```python
from build123d import *

# Parameters (mm, degrees)
CHAMFER_1_SIZE            = 0.2
FILLET_1_R                = 0.2
HOLE_WIZARD_4_0_4_1_D     = 4
HOLE_WIZARD_4_0_4_1_DEPTH = 2.5
HOLE_WIZARD_4_0_4_1_TIP   = 1.201721238
CUT_EXTRUDE_1_DEPTH       = 2.5
FILLET_2_R                = 0.2


with BuildPart() as part:
    # 草图1 → 旋转1 (revolve)
    with BuildSketch(Plane.XY):
        Polygon((0, 0), (0, 4.25), (5, 4.25), (5, 2.5), (40, 2.5), (40, 0), align=None)
    revolve(axis=Axis((0, 0, 0), (1, 0, 0)))

    # 倒角1
    chamfer_1_edges = [part.edges().sort_by_distance(p)[0] for p in [
        (40, -2.5, 0),
    ]]
    chamfer(chamfer_1_edges, length=CHAMFER_1_SIZE)

    # 圆角1
    fillet_1_edges = [part.edges().sort_by_distance(p)[0] for p in [
        (0, -4.25, 0),
    ]]
    fillet(fillet_1_edges, radius=FILLET_1_R)

    # Ø4.0 (4) 直径孔1
    with Locations(Plane.ZY):
        with Locations((0, 0)):
            Hole(HOLE_WIZARD_4_0_4_1_D / 2, depth=HOLE_WIZARD_4_0_4_1_DEPTH)
            with Locations((0, 0, -(HOLE_WIZARD_4_0_4_1_DEPTH + HOLE_WIZARD_4_0_4_1_TIP / 2))):  # 118° drill point
                Cone(0, HOLE_WIZARD_4_0_4_1_D / 2, HOLE_WIZARD_4_0_4_1_TIP, mode=Mode.SUBTRACT)

    # 草图2 → 切除-拉伸1 (cut)
    with BuildSketch(Plane.ZY):
        Polygon((0, -2.309401077), (2, -1.154700538), (2, 1.154700538), (0, 2.309401077), (-2, 1.154700538), (-2, -1.154700538), align=None)
    extrude(amount=-CUT_EXTRUDE_1_DEPTH, mode=Mode.SUBTRACT)

    # 圆角2
    fillet_2_edges = [part.edges().sort_by_distance(p)[0] for p in [
        (5, -2.5, 0),
    ]]
    fillet(fillet_2_edges, radius=FILLET_2_R)


solid = part.part
```
Build history of the part. All positions in model axes, mm. A direction names the side the tool comes from. Round coordinates to 2 decimals unless told otherwise and drop trailing zeros. Order: outer loops, then holes, each group sorted by start corner. A loop starts at its lowest first (then second) coordinate and runs counter-clockwise, first axis right, second up. Notation, with made-up numbers: (-27.5, 24.5) -> (-17.5, 24.5) arc R24 cw to (-17.5, 54.5) -> close; hole circle Ø4 at (-19.75, -9.75). An arc over 180 degrees is marked (long way). Answer in a Markdown table with one row per item.
1) Pin check, flat tips, straight feed: P1, Ø0.5, axis at y = 0.5, z = -1.5, coming from the -X side; P2, Ø0.5, axis at y = 1, z = 1.5, coming from the -X side; P3, Ø1, axis at y = -2.5, z = 2.5, coming from the +X side. Stop position of each tip, or through.
Values:
| item | result |
|---|---|
| P1 | x = 2.6 |
| P2 | x = 2.5 |
| P3 | x = 5 |
2) Which spindle directions (+Z, -Z, +X, -X, +Y, -Y) get a long thin tool onto all of the face, cutting with end or side? Do faces 1 (the cylindrical face through (22.74, -0.54, -2.44)), 2 (the flat face through (1.23, 1.74, -0.99)), 3 (the flat face through (40, 0, 0)). Say none if no direction does.
Values:
| item | result |
|---|---|
| face 1 | +X |
| face 2 | -X |
| face 3 | +Z, -Z, +X, +Y, -Y |
3) Mould opens along Y. For faces 4 (the flat face through (0, 2, -1)), 5 (the flat face through (1, 0, -2)), 6 (the flat face through (1.23, -1.74, 0.99)), 7 (the cylindrical face through (2.634, 2.285, 3.584)) say: released by +Y, released by -Y, zero draft, split by the parting line, or undercut.
Values:
| item | result |
|---|---|
| face 4 | zero draft |
| face 5 | undercut |
| face 6 | undercut |
| face 7 | split by the parting line |
4) Wall check: L1, parallel to X at y = 2.75, z = 1.75; L2, parallel to Z at x = 32.5, y = 1; L3, parallel to Z at x = 18, y = 0. Give the ranges that are in metal, low to high.
Values:
| item | result |
|---|---|
| L1 | 0 to 5 |
| L2 | -2.29 to 2.29 |
| L3 | -2.5 to 2.5 |
5) Band-saw the part on A-A on x = 21. Give the cut face in (y, z), and give its area (3 significant figures).
Values:
| item | result |
|---|---|
| outline | circle Ø5 at (0, 0) |
| area | 19.6 mm2 |
